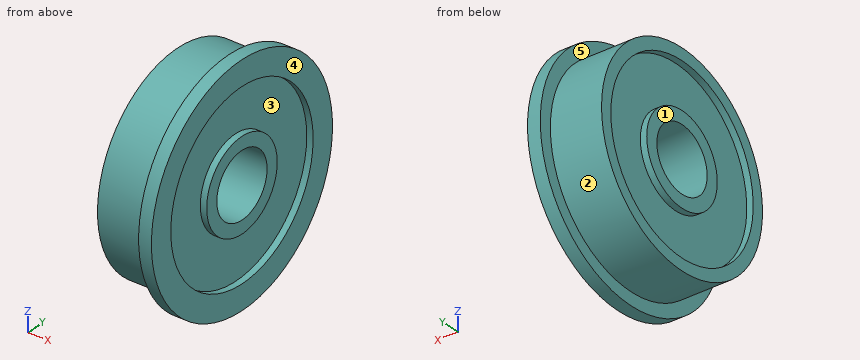
Autodesk Inventor part; units mm, degrees
ref_plane "YZ Plane" through (0, 0, 0) normal (1, 0, 0) x (0, 1, 0)
ref_plane "XZ Plane" through (0, 0, 0) normal (0, 1, 0) x (-1, 0, 0)
ref_plane "XY Plane" through (0, 0, 0) normal (0, 0, 1) x (1, 0, 0)
sketch "Эскиз1" plane through (0, 0, 0) normal (1, 0, 0) x (0, 1, 0)
  circle A0 centre (0, 0) radius 8
  circle A1 centre (0, 0) radius 2.5
  circle A2 centre (0, 0) radius 9
  circle A3 centre (0, 0) radius 7.0758
  circle A4 centre (0, 0) radius 3.5071
  dimension "d0" = 16
  dimension "d1" = 5
  dimension "d2" = 18
extrude "Выдавливание1" add sketch "Эскиз1" along normal mid plane 5 contours A0 | A4
extrude "Выдавливание2" add sketch "Эскиз1" along normal mid plane 4 contours A3
sketch "Эскиз2" plane through (2.5, 0, 0) normal (1, 0, 0) x (0, 0, -1)
  circle A0 centre (0, 0) radius 9
  circle A1 centre (0, 0) radius 8
  dimension "d7" = 18
  dimension "d8" = 16
extrude "Выдавливание3" add sketch "Эскиз2" against normal blind 1
properties part number "F625ZZ"
CAD build for the part. Positions are in the model's coordinates, mm. Face numbers are marked on the shaded views. A direction names the side the tool comes from. Coordinates: 2 decimals unless noted, no trailing zeros. Write each loop counter-clockwise with the first axis right and the second up, starting at its lowest first coordinate (ties: lowest second). Pieces come first, ordered by that corner, then holes. Notation, with made-up numbers: (52.25, 85.25) - (87.25, 85.25) arc R15 cw to (87.25, 113.25) - close; hole circle Ø10 at (-1, -25). An arc over 180 degrees is marked (long way). Use a Markdown table: item, result. Add a question column.
Item 1: 3-axis set-ups, long thin cutter, end or side, ignore diameter. For the marked faces 4 and 5: which of +Z, -Z, +X, -X, +Y, -Y reach the whole face in a straight line?
Item 2: Band-saw the part on A-A, the plane z = 0. Give the cut face in (x, y), and give its area (3 significant figures).
Item 3: Drill centre lines: L1, parallel to Z at x = 1.1, y = 0; L2, parallel to Z at x = -2.2, y = 0; L3, parallel to X at y = -3.75, z = -3.5. Where is each one in solid material? Low to high. Write a range as from..to.
Item 4: Flat gauge pins, fed straight in: pin 1 (6 mm diameter, centred on y = -5, z = 2.5, fed in from +X); pin 2 (4 mm diameter, centred on y = 0, z = 0, fed in from -X); pin 3 (1 mm diameter, centred on x = 0, z = -2, fed in from +Y); pin 4 (2 mm diameter, centred on x = -0.5, z = 6, fed in from +Y) (3 decimals). Where does each tip first touch, or does it go through?
Item 5: Band-saw the part on D-D, the plane y = 5.5. Give the cut face in (x, z).
Item 6: Band-saw the part on C-C, the plane x = 0.3. Give the cut face in (y, z), and give its area (3 significant figures).
Item 7: Mould opens along Z. For the marked faces 1, 2 and 3 say: pulls with the +Z half, pulls with the -Z half, needs draft (parallel to the pull), parting line crosses it, or undercut.
Numbers:
| question | item | result |
|---|---|---|
| 1 | face 4 | +Z, -Z, +X, +Y, -Y |
| 1 | face 5 | -X |
| 2 | outline | (-2.5, -8) - (1.5, -8) - (1.5, -9) - (2.5, -9) - (2.5, -7.08) - (2, -7.08) - (2, -3.51) - (2.5, -3.51) - (2.5, -2.5) - (-2.5, -2.5) - (-2.5, -3.51) - (-2, -3.51) - (-2, -7.08) - (-2.5, -7.08) - close; (-2.5, 2.5) - (2.5, 2.5) - (2.5, 3.51) - (2, 3.51) - (2, 7.08) - (2.5, 7.08) - (2.5, 9) - (1.5, 9) - (1.5, 8) - (-2.5, 8) - (-2.5, 7.08) - (-2, 7.08) - (-2, 3.51) - (-2.5, 3.51) - close |
| 2 | area | 49.9 mm2 |
| 3 | L1 | -8..-2.5, 2.5..8 |
| 3 | L2 | -8..-7.08, -3.51..-2.5, 2.5..3.51, 7.08..8 |
| 3 | L3 | -2..2 |
| 4 | pin 1 | x = 2.5 |
| 4 | pin 2 | through |
| 4 | pin 3 | y = 7.86 |
| 4 | pin 4 | y = 6.245 |
| 5 | outline | (-2.5, -5.81) - (1.5, -5.81) - (1.5, -7.12) - (2.5, -7.12) - (2.5, -4.45) - (2, -4.45) - (2, 4.45) - (2.5, 4.45) - (2.5, 7.12) - (1.5, 7.12) - (1.5, 5.81) - (-2.5, 5.81) - (-2.5, 4.45) - (-2, 4.45) - (-2, -4.45) - (-2.5, -4.45) - close |
| 6 | outline | circle Ø16 at (0, 0); hole circle Ø5 at (0, 0) |
| 6 | area | 181 mm2 |
| 7 | face 1 | needs draft |
| 7 | face 2 | parting line crosses it |
| 7 | face 3 | undercut |
